from build123d import *

# Parameters (mm, degrees)
BOSS_EXTRUDE3_DEPTH = 7
BOSS_EXTRUDE4_DEPTH = 1
BOSS_EXTRUDE5_DEPTH = 7
BOSS_EXTRUDE6_DEPTH = 3
BOSS_EXTRUDE7_START = -5
BOSS_EXTRUDE7_DEPTH = 2


with BuildPart() as part:
    # Sketch1 → Boss-Extrude3 (new body)
    with BuildSketch(Plane(origin=(0, 0, 0), x_dir=(1, 0, 0), z_dir=(0, 1, 0))):
        with BuildLine():
            Line((0.970071849, 4.904993436), (0.970071849, 3.843317436))
            ThreePointArc((0.970071849, 3.843317436), (0, -3.96385271), (-0.970071849, 3.843317436))
            Line((-0.970071849, 3.843317436), (-0.970071849, 4.904993436))
            ThreePointArc((-0.970071849, 4.904993436), (0, -5), (0.970071849, 4.904993436))
        make_face()
    extrude(amount=-BOSS_EXTRUDE3_DEPTH)

    # Sketch1<6> → Boss-Extrude4 (add)
    with BuildSketch(Plane(origin=(0, 0, 0), x_dir=(1, 0, 0), z_dir=(0, 1, 0))):
        with BuildLine():
            Line((0.970071849, 10.957141991), (0.970071849, 4.904993436))
            ThreePointArc((0.970071849, 4.904993436), (0, -5), (-0.970071849, 4.904993436))
            Line((-0.970071849, 4.904993436), (-0.970071849, 10.957141991))
            ThreePointArc((-0.970071849, 10.957141991), (0, -11), (0.970071849, 10.957141991))
        make_face()
    extrude(amount=-BOSS_EXTRUDE4_DEPTH)

    # Sketch1<7> → Boss-Extrude5 (add)
    with BuildSketch(Plane(origin=(0, 0, 0), x_dir=(1, 0, 0), z_dir=(0, 1, 0))):
        with BuildLine():
            ThreePointArc((-7.460787851, -9.503640297), (0, -12.082323214), (7.460787851, -9.503640297))
            Line((7.460787851, -9.503640297), (6.442669325, -8.915829292))
            ThreePointArc((6.442669325, -8.915829292), (0, -11), (-6.442669325, -8.915829292))
            Line((-6.442669325, -8.915829292), (-7.460787851, -9.503640297))
        make_face()
        with BuildLine():
            Line((10.942669325, -1.121600658), (11.960787851, -1.709411663))
            ThreePointArc((11.960787851, -1.709411663), (12.051901073, -0.856863332), (12.082323214, 0))
            ThreePointArc((12.082323214, 0), (10.008820827, 6.768015949), (4.5, 11.21305196))
            Line((4.5, 11.21305196), (4.5, 10.03742995))
            ThreePointArc((4.5, 10.03742995), (9.233092656, 5.979130372), (11, 0))
            ThreePointArc((11, 0), (10.985657982, -0.561532466), (10.942669325, -1.121600658))
        make_face()
        with BuildLine():
            ThreePointArc((-4.5, 11.21305196), (-10.46359884, 6.041161607), (-11.960787851, -1.709411663))
            Line((-11.960787851, -1.709411663), (-10.942669325, -1.121600658))
            ThreePointArc((-10.942669325, -1.121600658), (-9.526279442, 5.5), (-4.5, 10.03742995))
            Line((-4.5, 10.03742995), (-4.5, 11.21305196))
        make_face()
    extrude(amount=-BOSS_EXTRUDE5_DEPTH)

    # Sketch1<8> → Boss-Extrude6 (add)
    with BuildSketch(Plane(origin=(0, 0, 0), x_dir=(1, 0, 0), z_dir=(0, 1, 0))):
        with BuildLine():
            Line((11.960787851, -1.709411663), (10.942669325, -1.121600658))
            ThreePointArc((10.942669325, -1.121600658), (9.526279442, -5.5), (6.442669325, -8.915829292))
            Line((6.442669325, -8.915829292), (7.460787851, -9.503640297))
            ThreePointArc((7.460787851, -9.503640297), (10.46359884, -6.041161607), (11.960787851, -1.709411663))
        make_face()
        with BuildLine():
            Line((4.5, 10.03742995), (4.5, 11.21305196))
            ThreePointArc((4.5, 11.21305196), (2.766361636, 11.761368014), (0.970071849, 12.043317436))
            Line((0.970071849, 12.043317436), (0.970071849, 10.957141991))
            ThreePointArc((0.970071849, 10.957141991), (2.773425512, 10.644628267), (4.5, 10.03742995))
        make_face()
        with BuildLine():
            Line((-7.460787851, -9.503640297), (-6.442669325, -8.915829292))
            ThreePointArc((-6.442669325, -8.915829292), (-9.526279442, -5.5), (-10.942669325, -1.121600658))
            Line((-10.942669325, -1.121600658), (-11.960787851, -1.709411663))
            ThreePointArc((-11.960787851, -1.709411663), (-10.46359884, -6.041161607), (-7.460787851, -9.503640297))
        make_face()
        with BuildLine():
            Line((-0.970071849, 10.957141991), (-0.970071849, 12.043317436))
            ThreePointArc((-0.970071849, 12.043317436), (-2.766361636, 11.761368014), (-4.5, 11.21305196))
            Line((-4.5, 11.21305196), (-4.5, 10.03742995))
            ThreePointArc((-4.5, 10.03742995), (-2.773425512, 10.644628267), (-0.970071849, 10.957141991))
        make_face()
    extrude(amount=-BOSS_EXTRUDE6_DEPTH)

    # Sketch1<9> → Boss-Extrude7 (add)
    with BuildSketch(Plane(origin=(0, 0, 0), x_dir=(1, 0, 0), z_dir=(0, 1, 0)).offset(BOSS_EXTRUDE7_START)):
        with BuildLine():
            ThreePointArc((-9.944782921, -6.861765583), (-8.802462665, -8.276423459), (-7.460787851, -9.503640297))
            Line((-7.460787851, -9.503640297), (-6.442669325, -8.915829292))
            ThreePointArc((-6.442669325, -8.915829292), (-7.831805737, -7.724171082), (-9.004127392, -6.31867786))
            Line((-9.004127392, -6.31867786), (-9.944782921, -6.861765583))
        make_face()
        with BuildLine():
            ThreePointArc((10.91485477, -5.181551853), (11.568824301, -3.484944554), (11.960787851, -1.709411663))
            Line((11.960787851, -1.709411663), (10.942669325, -1.121600658))
            ThreePointArc((10.942669325, -1.121600658), (10.605231248, -2.920457185), (9.974199241, -4.638464131))
            Line((9.974199241, -4.638464131), (10.91485477, -5.181551853))
        make_face()
        with BuildLine():
            Line((-0.970071849, 10.957141991), (-0.970071849, 12.043317436))
            ThreePointArc((-0.970071849, 12.043317436), (-2.766361636, 11.761368014), (-4.5, 11.21305196))
            Line((-4.5, 11.21305196), (-4.5, 10.03742995))
            ThreePointArc((-4.5, 10.03742995), (-2.773425512, 10.644628267), (-0.970071849, 10.957141991))
        make_face()
    extrude(amount=-BOSS_EXTRUDE7_DEPTH)


solid = part.part
Could you check a few things on this model? Use its own coordinates, in mm. A direction names the side the tool comes from. Coordinates: 2 decimals unless noted, no trailing zeros. Loops run counter-clockwise (first coordinate to the right, second up) from the corner with the lowest first, then second, coordinate; pieces in that order, holes last.
1. Imagine slicing it at D-D (z = -8.5). Please give me the cut outline in (x, y), and give its area (3 significant figures).
2. Imagine slicing it at A-A (y = -1.75). Please give me the cut outline in (x, z) (3 decimals), and give its area (3 significant figures).
3. For faces 1 (the face through (-0.97, -6, -11.5)), 2 (the face through (3, -3, -11)), 3 (the face through (2, -1, 5)), 4 (the face through (-8, -5, 8)), 5 (the face through (-3, -5, -11)), which set-ups out of +Z, -Z, +X, -X, +Y, -Y let a thin tool reach every point of the face, with its end or its side?
4. Imagine slicing it at B-B (y = -5.75). Please give me the cut outline in (x, z) (3 decimals), and give its area (3 significant figures).
5. For P1, Ø2, axis at y = -2, z = -7, coming from the -X side; P2, Ø1, axis at x = 11.5, z = 2.5, coming from the +Y side; P3, Ø4, axis at x = -3, y = -5, coming from the -Z side; P4, Ø3, axis at y = -2, z = -2, coming from the -X side, each with a flat end and sliding along its axis, tell me the tip position at first contact or that it passes through.
6. I need wall thicknesses on L1, parallel to Z at x = 0, y = -3.25; L2, parallel to X at y = -1.5, z = -1.5; L3, parallel to X at y = -3.25, z = -2.5. Which ranges of each line are inside material? Lowest first, please.
7. We'd pull the mould along X, two halves only. Please class faces 6 (the face through (0.97, -0.6, -7.4)), 7 (the face through (11, -7, -4)), 8 (the face through (-9.468, -5.986, 6.586)): released by +X, released by -X, zero draft, split by the parting line, or undercut.
8. Imagine slicing it at C-C (x = 0). Please give me the cut outline in (y, z).
Computed values:
1. outline: (-8.59, -7) - (-6.98, -7) - (-6.98, -1) - (-0.97, -1) - (-0.97, 0) - (-8.59, 0) - close; (0.97, -1) - (6.98, -1) - (6.98, -7) - (8.59, -7) - (8.59, 0) - (0.97, 0) - close
1. area: 34.5 mm2
2. outline: (-0.97, -12.043) - (-0.97, -10.957) arc R11 cw (long way) to (0.97, -10.957) - (0.97, -12.043) arc R12.082 ccw (long way) to start; (-0.97, -4.905) - (-0.97, -3.843) arc R3.964 cw (long way) to (0.97, -3.843) - (0.97, -4.905) arc R5 ccw (long way) to start
2. area: 104 mm2
3. face 1: -Z, +Y, -Y
3. face 2: -Z, -Y
3. face 3: -Y
3. face 4: -X
3. face 5: -Z
4. outline: (-11.961, 1.709) arc R12.082 ccw to (-0.97, -12.043) - (-0.97, -10.957) arc R11 cw to (-10.943, 1.122) - close; (-9.945, 6.862) - (-9.004, 6.319) arc R11 cw to (6.443, 8.916) - (7.461, 9.504) arc R12.082 ccw to start; (-0.97, -4.905) - (-0.97, -3.843) arc R3.964 cw (long way) to (0.97, -3.843) - (0.97, -4.905) arc R5 ccw (long way) to start; (4.5, -11.213) arc R12.082 ccw to (10.915, 5.182) - (9.974, 4.638) arc R11 cw to (4.5, -10.037) - close
4. area: 87.5 mm2
5. P1: stops at x = -10.49
5. P2: stops at y = 0
5. P3: stops at z = -12.04
5. P4: stops at x = -12.07
6. L1: z = 3.96 to 5, 11 to 12.08
6. L2: x = -11.99 to -10.9, -4.77 to -3.67, 3.67 to 4.77, 10.9 to 11.99
6. L3: x = -11.82 to -10.71, -4.33 to -3.08, 3.08 to 4.33, 10.71 to 11.82
7. face 6: undercut
7. face 7: zero draft
7. face 8: released by -X
8. outline: (-7, 3.96) - (0, 3.96) - (0, 12.08) - (-7, 12.08) - (-7, 11) - (-1, 11) - (-1, 5) - (-7, 5) - close
